Work out the finished part from the listing and answer in its coordinate system (mm). Face numbers are marked on the shaded views. A direction names the side the tool comes from. Coordinates: 2 decimals unless noted, no trailing zeros. Order: outer loops, then holes, each group sorted by start corner. A loop starts at its lowest first (then second) coordinate and runs counter-clockwise, first axis right, second up. Notation, with made-up numbers: M 24.5,48 L 65.5,48 A31 ccw 65.5,72 Z; hole C 11.25,32.5 d6. An arc over 180 degrees is marked long. Answer in a Markdown table with one row per item. Add a question column.
Item 1: The part is cut by section B-B (x = 0). Write down the section's boundary in (y, z) (3 decimals), then the cut area to 3 significant figures.
Item 2: The mould has two halves that part along Z. Classify the marked faces 1, 2, 3 and 4: released by +Z, released by -Z, zero draft, split by the parting line, or undercut.
Item 3: Consider line 1 (Y direction, x = -1, z = 2.25); line 2 (Y direction, x = 0.75, z = 0); line 3 (Z direction, x = 0.5, y = 6.5). Determine where each line is inside the solid, lowest interval first. Write a range as from..to.
Item 4: The part is cut by section C-C (z = 0). Write down the section's boundary in (x, y) (3 decimals).
Item 5: The part is cut by section D-D (x = 2.1). Write down the section's boundary in (y, z).
Item 6: Flat-ended cylindrical pins translate along their axes: pin 1 Ø0.5 at (y, z) = (-2.5, -2.5) entering from -X; pin 2 Ø0.7 at (y, z) = (-1.5, -2.5) entering from +X; pin 3 Ø0.5 at (x, z) = (-2, 2) entering from +Y; pin 4 Ø1.9 at (x, z) = (0.5, 1.5) entering from -Y. Find the tip coordinate at first contact, or state that the pin passes through.
Item 7: Which of the six approach directions +Z, -Z, +X, -X, +Y, -Y give full straight-line access (tool end or side, diameter ignored) to the marked faces 5 and 6?
Item 8: The part is cut by section A-A (y = -0.25). Write down the section's boundary in (x, z).
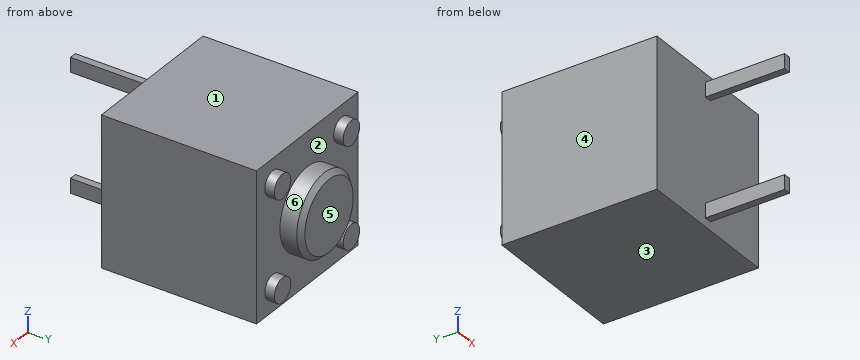
Autodesk Inventor part; units mm, degrees
ref_plane "YZ Plane" through (0, 0, 0) normal (1, 0, 0) x (0, 1, 0)
ref_plane "XZ Plane" through (0, 0, 0) normal (0, 1, 0) x (-1, 0, 0)
ref_plane "XY Plane" through (0, 0, 0) normal (0, 0, 1) x (1, 0, 0)
sketch "Sketch1" plane through (0, 0, 0) normal (0, 1, 0) x (-1, 0, 0)
  line L0 (3.1, 3.1) -> (-3.1, 3.1)
  line L1 (-3.1, 3.1) -> (-3.1, -3.1)
  line L2 (-3.1, -3.1) -> (3.1, -3.1)
  line L3 (3.1, -3.1) -> (3.1, 3.1)
  line L4 (4.34, 0) -> (-4.34, 0) construction
  line L5 (0, -4.34) -> (0, 4.34) construction
  point P0 (0, 0)
  dimension "d0" = 6.2
  dimension "d1" = 6.2
extrude "Extrusion1" add sketch "Sketch1" along normal blind 6.45
sketch "Sketch2" plane through (0, 6.45, 0) normal (0, 1, 0) x (1, 0, 0)
  circle A0 centre (-2.1, -2.1) radius 0.5
  circle A1 centre (-2.1, 2.1) radius 0.5
  circle A2 centre (2.1, 2.1) radius 0.5
  circle A3 centre (2.1, -2.1) radius 0.5
  line L0 (-3.1, -3.1) -> (3.1, -3.1)
  line L1 (-3.1, 3.1) -> (-3.1, -3.1)
  line L2 (3.1, 3.1) -> (-3.1, 3.1)
  line L3 (3.1, -3.1) -> (3.1, 3.1)
  point P0 (0, 0)
  dimension "d4" = 1
  dimension "d5" = 1
  dimension "d6" = 1
  dimension "d7" = 1
  dimension "d8" = 1
  dimension "d9" = 1
  dimension "d10" = 1
  dimension "d11" = 1
extrude "Extrusion2" add sketch "Sketch2" along normal blind 0.4 contours A0 | A1 | A2 | A3
sketch "Sketch3" plane through (0, 6.45, 0) normal (0, 1, 0) x (1, 0, 0)
  circle A0 centre (0, 0) radius 1.675
  dimension "d14" = 3.35
extrude "Extrusion3" add sketch "Sketch3" along normal blind 0.9
chamfer "Chamfer1" distance 0.2 angle 45 1 edges at (-1.675, 7.35, 0)
sketch "Sketch4" plane through (0, 0, 0) normal (1, 0, 0) x (0, 1, 0)
  line L0 (0, 3.1) -> (0, -3.1)
  line L1 (0, 2.75) -> (-3.3, 2.75)
  line L2 (-3.3, 2.75) -> (-3.3, 2.15)
  line L3 (-3.3, 2.15) -> (0, 2.15)
  line L4 (0, -2.15) -> (-3.3, -2.15)
  line L5 (-3.3, -2.15) -> (-3.3, -2.75)
  line L6 (-3.3, -2.75) -> (0, -2.75)
  line L7 (-3.96, 0) -> (0.66, 0)
  point P0 (0, 0)
  dimension "d20" = 5.5
  dimension "d21" = 0.6
  dimension "d22" = 0.6
  dimension "d23" = 3.3
extrude "Extrusion4" add sketch "Sketch4" along normal mid plane 0.3
properties part number "6mm_switch"
Reply:
| question | item | result |
|---|---|---|
| 1 | outline | M -3.3,-2.75 L 0,-2.75 L 0,-3.1 L 6.45,-3.1 L 6.45,-1.675 L 7.15,-1.675 L 7.35,-1.475 L 7.35,1.475 L 7.15,1.675 L 6.45,1.675 L 6.45,3.1 L 0,3.1 L 0,2.75 L -3.3,2.75 L -3.3,2.15 L 0,2.15 L 0,-2.15 L -3.3,-2.15 Z |
| 1 | area | 46.9 mm2 |
| 2 | face 1 | released by +Z |
| 2 | face 2 | undercut |
| 2 | face 3 | released by -Z |
| 2 | face 4 | zero draft |
| 3 | line 1 | y = 0..6.45 |
| 3 | line 2 | y = 0..7.35 |
| 3 | line 3 | z = -1.6..1.6 |
| 4 | outline | M -3.1,0 L 3.1,0 L 3.1,6.45 L 1.675,6.45 L 1.675,7.15 L 1.475,7.35 L -1.475,7.35 L -1.675,7.15 L -1.675,6.45 L -3.1,6.45 Z |
| 5 | outline | M 0,-3.1 L 6.45,-3.1 L 6.45,-2.6 L 6.85,-2.6 L 6.85,-1.6 L 6.45,-1.6 L 6.45,1.6 L 6.85,1.6 L 6.85,2.6 L 6.45,2.6 L 6.45,3.1 L 0,3.1 Z |
| 6 | pin 1 | stops at x = -0.15 |
| 6 | pin 2 | stops at x = 0.15 |
| 6 | pin 3 | stops at y = 6.85 |
| 6 | pin 4 | stops at y = -3.3 |
| 7 | face 5 | +Z, -Z, +X, -X, +Y |
| 7 | face 6 | +Y |
| 8 | outline | M -0.15,-2.75 L 0.15,-2.75 L 0.15,-2.15 L -0.15,-2.15 Z; M -0.15,2.15 L 0.15,2.15 L 0.15,2.75 L -0.15,2.75 Z |
